Design review of the part shown in the three views and the two pictorial views. Dimensions are in mm from the part's minimum x, y and z. Coordinates: 2 decimals unless noted, no trailing zeros. Write each loop counter-clockwise with the first axis right and the second up, starting at its lowest first coordinate (ties: lowest second). Pieces come first, ordered by that corner, then holes. Notation, with made-up numbers: (36.25, 42.25) -> (51.25, 42.25) arc R31 cw to (51.25, 71.25) -> close; hole circle Ø5 at (-37.75, 40). An arc over 180 degrees is marked (long way). Write item = value, one per line. Start each with the question number.
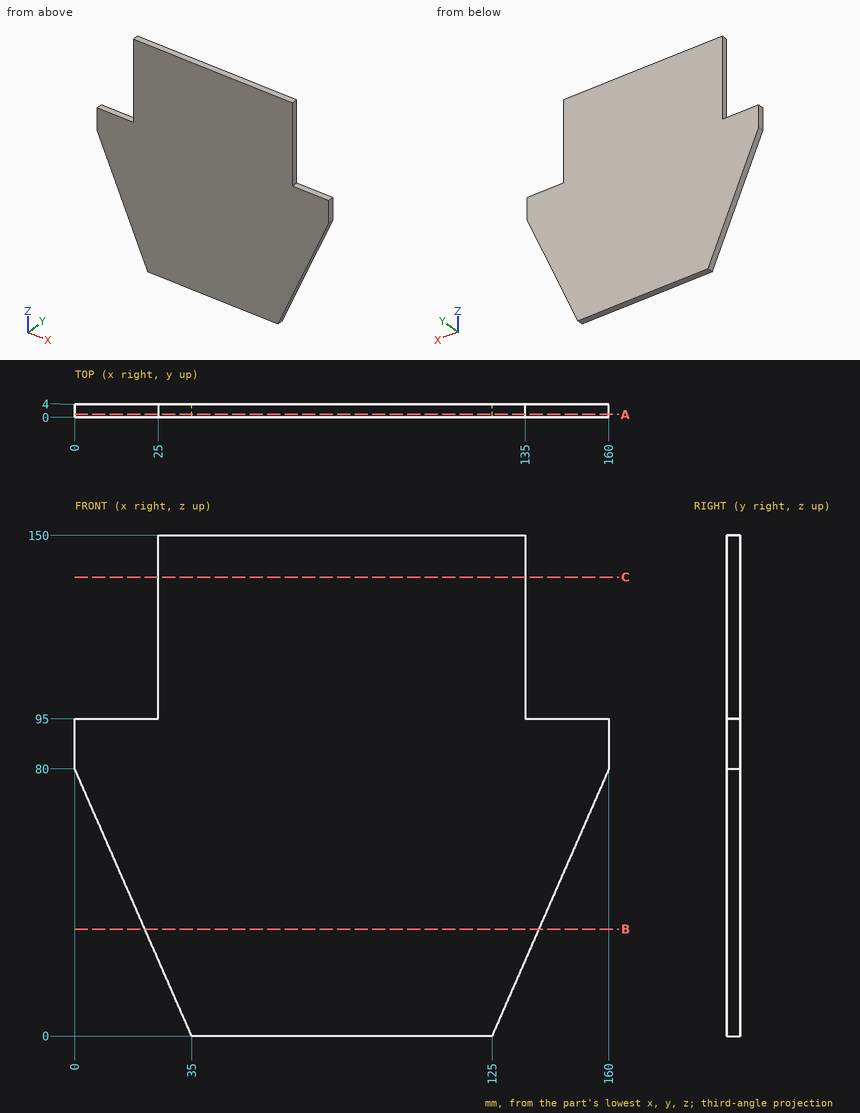
(1) Take a section at C-C, the plane z = 137.5. State the section outline as (x, y) points.
(2) For line 1 (X direction, y = 2.45, z = 103); line 2 (Z direction, x = 132.5, y = 0.25); line 3 (X direction, y = 2.1, z = 10.5), list the stretches that pass through material, from the lowest coordinate up.
(3) Take a section at A-A, the plane y = 0.9. State the section outline as (x, z) points.
(4) For pin 1 Ø2 at (x, y) = (145.5, 2) entering from +Z; pin 2 Ø1.2 at (y, z) = (3, 126.5) entering from -X; pin 3 Ø10 at (x, z) = (129.5, 52.5) entering from -Y, all flat-tipped, find the tip position at first contact; note any pin that passes through.
(5) Take a section at B-B, the plane z = 32. State the section outline as (x, y) points, then the cut area to 3 significant figures.
Report:
q1.outline = (25, 0) -> (135, 0) -> (135, 4) -> (25, 4) -> close
q2.line_1 = 25 to 135
q2.line_2 = 17.14 to 150
q2.line_3 = 30.41 to 129.59
q3.outline = (0, 80) -> (35, 0) -> (125, 0) -> (160, 80) -> (160, 95) -> (135, 95) -> (135, 150) -> (25, 150) -> (25, 95) -> (0, 95) -> close
q4.pin_1 = 95
q4.pin_2 = 25
q4.pin_3 = 0
q5.outline = (21, 0) -> (139, 0) -> (139, 4) -> (21, 4) -> close
q5.area = 472 mm2
